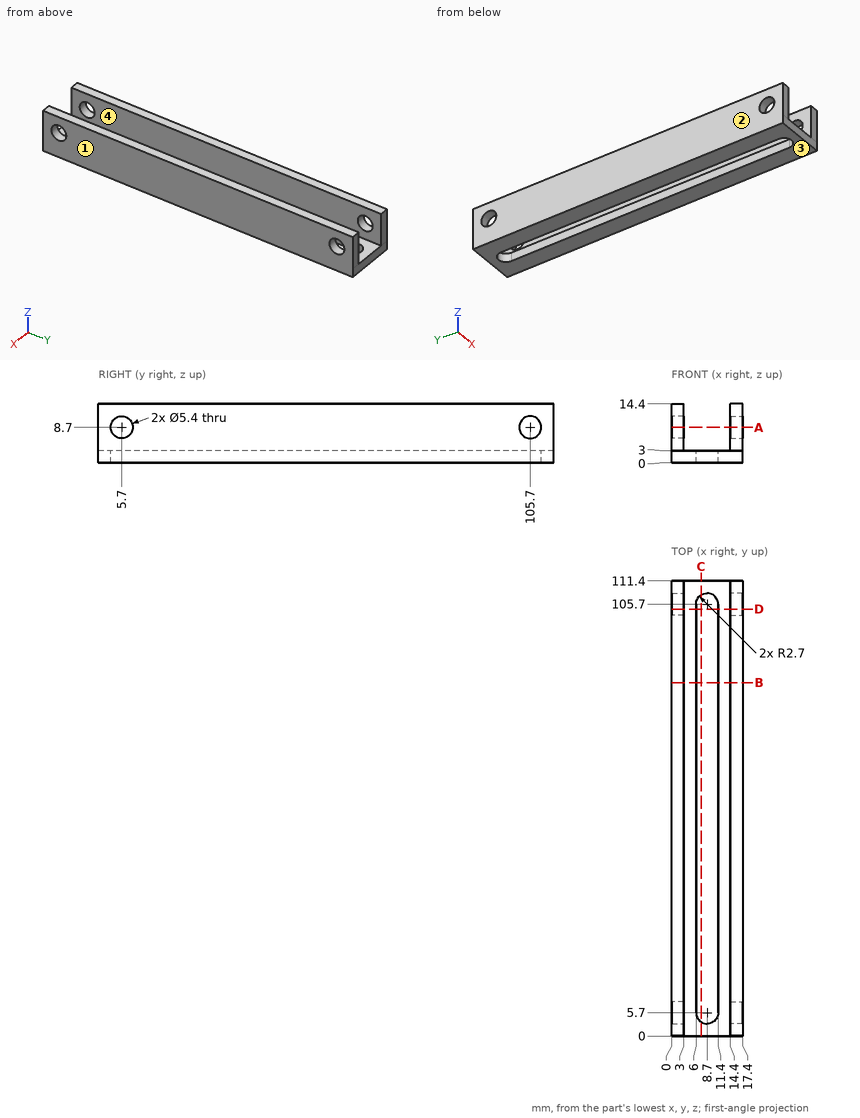
Study the drawing (mm; zero at the part's minimum x, y, z) and answer. Give positions to 0.01 mm unless a question says otherwise; leave off trailing zeros. Write each loop counter-clockwise with the first axis right and the second up, starting at its lowest first coordinate (ties: lowest second). Pieces come first, ordered by that corner, then holes. Notation, with made-up numbers: (39.25, 15) -> (75.25, 15) arc R25 ccw to (75.25, 33) -> close; hole circle Ø8 at (-39, -32). An arc over 180 degrees is marked (long way). Write item = value, one per line.
Q1. Section C-C on x = 7.25 is taken. Determine the outline of the cut face in (y, z).
Computed values:
outline = (0, 0) -> (3.42, 0) -> (3.42, 3) -> (0, 3) -> close; (107.98, 0) -> (111.4, 0) -> (111.4, 3) -> (107.98, 3) -> close
Q2. Consider line 1 along X through (y, z) = (92, 9); line 2 along X through (y, z) = (47, 1.25); line 3 along Z through (x, y) = (13, 38). Determine where each line is inside the solid, lowest interval first.
Computed values:
line_1 = 0 to 3, 14.4 to 17.4
line_2 = 0 to 6, 11.4 to 17.4
line_3 = 0 to 3
Q3. Section B-B on y = 86.5 is taken. Determine the outline of the cut face in (x, z).
Computed values:
outline = (0, 0) -> (6, 0) -> (6, 3) -> (3, 3) -> (3, 14.4) -> (0, 14.4) -> close; (11.4, 0) -> (17.4, 0) -> (17.4, 14.4) -> (14.4, 14.4) -> (14.4, 3) -> (11.4, 3) -> close
Q4. For a pull along X with two mould halves and no side action, classify the marked faces 1, 2, 3 and 4 as pulls with the +X half, pulls with the -X half, needs draft (parallel to the pull), parting line crosses it, or undercut.
Computed values:
face_1 = pulls with the +X half
face_2 = pulls with the -X half
face_3 = needs draft
face_4 = undercut
Q5. Section D-D on y = 104.5 is taken. Determine the outline of the cut face in (x, z), and give its area (3 significant figures).
Computed values:
outline = (0, 0) -> (6, 0) -> (6, 3) -> (3, 3) -> (3, 6.28) -> (0, 6.28) -> close; (0, 11.12) -> (3, 11.12) -> (3, 14.4) -> (0, 14.4) -> close; (11.4, 0) -> (17.4, 0) -> (17.4, 6.28) -> (14.4, 6.28) -> (14.4, 3) -> (11.4, 3) -> close; (14.4, 11.12) -> (17.4, 11.12) -> (17.4, 14.4) -> (14.4, 14.4) -> close
area = 75.4 mm^2
Q6. Section A-A on z = 8.7 is taken. Determine the outline of the cut face in (x, y), and give its area (3 significant figures).
Computed values:
outline = (0, 0) -> (3, 0) -> (3, 3) -> (0, 3) -> close; (0, 8.4) -> (3, 8.4) -> (3, 103) -> (0, 103) -> close; (0, 108.4) -> (3, 108.4) -> (3, 111.4) -> (0, 111.4) -> close; (14.4, 0) -> (17.4, 0) -> (17.4, 3) -> (14.4, 3) -> close; (14.4, 8.4) -> (17.4, 8.4) -> (17.4, 103) -> (14.4, 103) -> close; (14.4, 108.4) -> (17.4, 108.4) -> (17.4, 111.4) -> (14.4, 111.4) -> close
area = 604 mm^2
